from build123d import *

# Parameters (mm, degrees)
SKETCH1_R                             = 41.656
SKETCH1_R_2                           = 38.227
BOSS_EXTRUDE1_DEPTH                   = 414.3375
CUT_EXTRUDE1_REACH                    = 428.171
CUT_EXTRUDE1_END_RADIUS               = 38.227
SKETCH2_R                             = 1.778
CIRPATTERN1_COUNT                     = 3
PRESSURE_EQUALIZATION_HOLE_REACH      = 428.171
PRESSURE_EQUALIZATION_HOLE_END_RADIUS = 38.227
SKETCH3_R                             = 2.38125
CIRPATTERN2_COUNT                     = 3
CUT_EXTRUDE3_REACH                    = 426.678
CUT_EXTRUDE3_END_RADIUS               = 38.227
SKETCH4_R                             = 1.7859375
CIRPATTERN3_COUNT                     = 3


with BuildPart() as part:
    # Sketch1 → Boss-Extrude1 (new body)
    with BuildSketch(Plane(origin=(0, 0, 0), x_dir=(1, 0, 0), z_dir=(0, 1, 0))):
        with Locations(Location((0, 0, 0), (0, 0, 270))):
            Circle(SKETCH1_R)
        with Locations(Location((0, 0, 0), (0, 0, 270))):
            Circle(SKETCH1_R_2, mode=Mode.SUBTRACT)
    extrude(amount=BOSS_EXTRUDE1_DEPTH)

    # Cut-Extrude1: up to this cylinder (the profile starts outside it)
    cut_extrude1_end = Plane(origin=(0, 76.2, 0), z_dir=(0, -1, 0)) * Cylinder(CUT_EXTRUDE1_END_RADIUS, 933.796, mode=Mode.PRIVATE)
    # Sketch2 → Cut-Extrude1 (cut, up to the surface)
    with BuildSketch(Plane(origin=(-20.828, 0, 36.07515422), x_dir=(0, -1, 0), z_dir=(-0.499999999999998, 0, 0.8660254037844398)), mode=Mode.PRIVATE) as cut_extrude1_sk1:
        with Locations(Location((-76.2, 0, 0), (0, 0, 90))):
            Circle(SKETCH2_R)
    cut_extrude1_tool1 = extrude(cut_extrude1_sk1.sketch, amount=-CUT_EXTRUDE1_REACH, mode=Mode.PRIVATE) - cut_extrude1_end
    cut_extrude1 = cut_extrude1_tool1.solids().sort_by_distance((-20.828, 76.2, 36.075154))[0]
    add(cut_extrude1, mode=Mode.SUBTRACT)

    # CirPattern1: Cut-Extrude1 ×3 about axis
    cirpattern1_axis = Axis((0, -7.62, 0), (0, 1, 0))
    for i in range(1, CIRPATTERN1_COUNT):
        add(cut_extrude1.rotate(cirpattern1_axis, i * 360 / CIRPATTERN1_COUNT), mode=Mode.SUBTRACT)

    # Pressure Equalization Hole: up to this cylinder (the profile starts outside it)
    pressure_equalization_hole_end = Plane(origin=(0, 207.16875, 0), z_dir=(0, -1, 0)) * Cylinder(PRESSURE_EQUALIZATION_HOLE_END_RADIUS, 933.796, mode=Mode.PRIVATE)
    # Sketch3 → Pressure Equalization Hole (cut, up to the surface)
    with BuildSketch(Plane(origin=(-20.828, 0, 36.07515422), x_dir=(0, -1, 0), z_dir=(-0.499999999999998, 0, 0.8660254037844398)), mode=Mode.PRIVATE) as pressure_equalization_hole_sk1:
        with Locations(Location((-207.16875, 0, 0), (0, 0, 90))):
            Circle(SKETCH3_R)
    pressure_equalization_hole_tool1 = extrude(pressure_equalization_hole_sk1.sketch, amount=-PRESSURE_EQUALIZATION_HOLE_REACH, mode=Mode.PRIVATE) - pressure_equalization_hole_end
    pressure_equalization_hole = pressure_equalization_hole_tool1.solids().sort_by_distance((-20.828, 207.16875, 36.075154))[0]
    add(pressure_equalization_hole, mode=Mode.SUBTRACT)

    # CirPattern2: Pressure Equalization Hole ×3 about axis
    cirpattern2_axis = Axis((0, -7.62, 0), (0, 1, 0))
    for i in range(1, CIRPATTERN2_COUNT):
        add(pressure_equalization_hole.rotate(cirpattern2_axis, i * 360 / CIRPATTERN2_COUNT), mode=Mode.SUBTRACT)

    # Cut-Extrude3: up to this cylinder (the profile starts outside it)
    cut_extrude3_end = Plane(origin=(0, 380.5301, 0), z_dir=(0, -1, 0)) * Cylinder(CUT_EXTRUDE3_END_RADIUS, 930.81, mode=Mode.PRIVATE)
    # Sketch4 → Cut-Extrude3 (cut, up to the surface)
    with BuildSketch(Plane(origin=(41.656, 0, 0), x_dir=(0, -1, 0), z_dir=(-1, 0, 0)), mode=Mode.PRIVATE) as cut_extrude3_sk1:
        with Locations(Location((-380.5301, 0, 0), (0, 0, 270))):
            Circle(SKETCH4_R)
    cut_extrude3_tool1 = extrude(cut_extrude3_sk1.sketch, amount=CUT_EXTRUDE3_REACH, mode=Mode.PRIVATE) - cut_extrude3_end
    cut_extrude3 = cut_extrude3_tool1.solids().sort_by_distance((41.656, 380.5301, 0))[0]
    add(cut_extrude3, mode=Mode.SUBTRACT)

    # CirPattern3: Cut-Extrude3 ×3 about axis
    cirpattern3_axis = Axis((0, -7.62, 0), (0, 1, 0))
    for i in range(1, CIRPATTERN3_COUNT):
        add(cut_extrude3.rotate(cirpattern3_axis, i * 360 / CIRPATTERN3_COUNT), mode=Mode.SUBTRACT)


solid = part.part
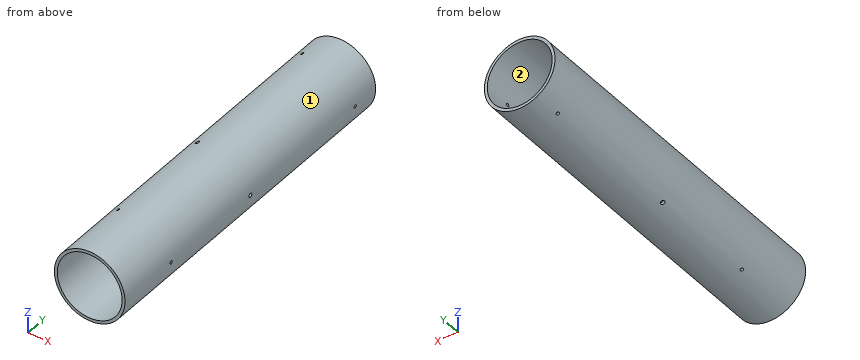
Can you work these out from the model? Positions are in its coordinate system, mm. Face numbers are marked on the shaded views. Coordinates: 2 decimals unless noted, no trailing zeros. Order: outer loops, then holes, each group sorted by start corner. A loop starts at its lowest first (then second) coordinate and runs counter-clockwise, first axis right, second up. Notation, with made-up numbers: (52.5, 14) - (79.5, 14) arc R24 ccw to (79.5, 39) - close; hole circle Ø11 at (50, -30.75). An arc over 180 degrees is marked (long way). Answer as a JSON object with one key per item and string values. Group by question number.
Q1. Imagine slicing it at A-A (x = 0). Please give me the cut outline in (y, z).
Q2. I need wall thicknesses on line 1 (Y direction, x = 39, z = 0); line 2 (X direction, y = 340.5, z = 2); line 3 (Z direction, x = 15, y = 31). Which ranges of each line are inside material? Lowest first, please. Write a range as from..to.
Q3. Imagine slicing it at C-C (y = 322). Please give me the cut outline in (x, z).
Q4. Imagine slicing it at B-B (z = -19.5). Please give me the cut outline in (x, y), and give its area (3 significant figures).
Q5. We'd pull the mould along Z, two halves only. Please class the marked faces 1 and 2: +Z half, -Z half, draft (parallel to the pull), parting line (faces both ways), or undercut.
Q6. Will these pins go through, and if not, where does the flat tip stop? P1, Ø5, axis at y = 111, z = -16, coming from the -X side; P2, Ø8, axis at x = 30.5, y = 77, coming from the +Z side; P3, Ø3, axis at y = 380.53, z = 0, coming from the +X side.
Determined:
{
 "1": {"outline": "(0, -41.66) - (414.34, -41.66) - (414.34, -38.23) - (0, -38.23) - close; (0, 38.23) - (414.34, 38.23) - (414.34, 41.66) - (0, 41.66) - close"},
 "2": {"line 1": "y = 0..74.42, 77.98..204.79, 209.55..378.74, 382.32..414.34", "line 2": "x = -41.61..-38.17, 38.17..41.61", "line 3": "z = -38.86..-35.16, 35.16..38.86"},
 "3": {"outline": "circle Ø83.31 at (0, 0); hole circle Ø76.45 at (0, 0)"},
 "4": {"outline": "(-36.81, 0) - (-32.88, 0) - (-32.88, 414.34) - (-36.81, 414.34) - close; (32.88, 0) - (36.81, 0) - (36.81, 414.34) - (32.88, 414.34) - close", "area": "3,260 mm2"},
 "5": {"face 1": "parting line", "face 2": "undercut"},
 "6": {"P1": "stops at x = -39.41", "P2": "stops at z = 32.14", "P3": "stops at x = -38.2"}
}
